Design review of the part built by this model. Coordinates are the model's own, in mm. A direction names the side the tool comes from. Coordinates: 2 decimals unless noted, no trailing zeros. Loops run counter-clockwise (first coordinate to the right, second up) from the corner with the lowest first, then second, coordinate; pieces in that order, holes last. Notation, with made-up numbers: (69, 50.5) -> (126, 50.5) arc R23 ccw to (126, 82.5) -> close; hole circle Ø10 at (27.5, 32.25). An arc over 180 degrees is marked (long way). Answer as a JSON object with one key per item and string values.
```python
from build123d import *

# Parameters (mm, degrees)
SKETCH2_W           = 33.5
SKETCH2_H           = 26
BOSS_EXTRUDE2_DEPTH = 5
FILLET2_R           = 5


with BuildPart() as part:
    # Sketch2 → Boss-Extrude2 (new body)
    # profile 1 of 4: a face of its own
    with BuildSketch(Plane.XY):
        Polygon((-19, -37.5), (-19, -63.5), (-5, -63.5), (-5, -58.5), (5, -58.5), (5, -63.5), (19, -63.5), (19, 63.5), (5, 63.5), (5, 58.5), (-5, 58.5), (-5, 63.5), (-19, 63.5), (-19, 37.5), (-52.5, 37.5), (-52.5, 32.5), (-67.5, 32.5), (-67.5, 37.5), (-75, 37.5), (-75, 0), (-75, -37.5), (-67.5, -37.5), (-67.5, -32.5), (-52.5, -32.5), (-52.5, -37.5), align=None)
    # profile 2 of 4: a face of its own
    with BuildSketch(Plane.XY):
        with Locations((-35.75, 50.5)):
            Rectangle(SKETCH2_W, SKETCH2_H)
        with BuildLine():
            Line((-44.75, 53.5), (-26.75, 53.5))
            ThreePointArc((-26.75, 53.5), (-20.75, 47.5), (-26.75, 41.5))
            Line((-26.75, 41.5), (-44.75, 41.5))
            ThreePointArc((-44.75, 41.5), (-50.75, 47.5), (-44.75, 53.5))
        make_face(mode=Mode.SUBTRACT)
    # profile 3 of 4: a face of its own
    with BuildSketch(Plane.XY):
        with Locations((-35.75, -50.5)):
            Rectangle(SKETCH2_W, SKETCH2_H)
        with BuildLine():
            ThreePointArc((-26.75, -53.5), (-20.75, -47.5), (-26.75, -41.5))
            Line((-26.75, -41.5), (-44.75, -41.5))
            ThreePointArc((-44.75, -41.5), (-50.75, -47.5), (-44.75, -53.5))
            Line((-44.75, -53.5), (-26.75, -53.5))
        make_face(mode=Mode.SUBTRACT)
    # profile 4 of 4: a face of its own
    with BuildSketch(Plane.XY):
        Polygon((-19, -37.5), (-19, -63.5), (-5, -63.5), (-5, -58.5), (5, -58.5), (5, -63.5), (19, -63.5), (19, 63.5), (5, 63.5), (5, 58.5), (-5, 58.5), (-5, 63.5), (-19, 63.5), (-19, 37.5), (-52.5, 37.5), (-52.5, 32.5), (-67.5, 32.5), (-67.5, 37.5), (-75, 37.5), (-75, 0), (-75, -37.5), (-67.5, -37.5), (-67.5, -32.5), (-52.5, -32.5), (-52.5, -37.5), align=None)
    extrude(amount=BOSS_EXTRUDE2_DEPTH)

    # Fillet2
    fillet2_edges = [part.edges().sort_by_distance(p)[0] for p in [
        (19, 63.5, 2.5),
        (19, -63.5, 2.5),
        (-52.5, -63.5, 2.5),
        (-75, -37.5, 2.5),
        (-75, 37.5, 2.5),
        (-52.5, 63.5, 2.5),
    ]]
    fillet(fillet2_edges, radius=FILLET2_R)


solid = part.part
```
1) The part is to be moulded in two halves that separate along Y. For faces 5 (the flat face through (0, 58.5, 2)), 6 (the cylindrical face through (-50.75, -47.37, 2.46)), 7 (the flat face through (19, -1, 2)), say which applies: pulls with the +Y half, pulls with the -Y half, needs draft (parallel to the pull), parting line crosses it, or undercut.
Completed:
{"face 5": "pulls with the +Y half", "face 6": "undercut", "face 7": "needs draft"}
2) Add section B-B, the plane y = 47.5. Give the boundary of the cut face in (x, z), and give its area (4 significant figures).
Completed:
{"outline": "(-52.5, 0) -> (-50.75, 0) -> (-50.75, 5) -> (-52.5, 5) -> close; (-20.75, 0) -> (19, 0) -> (19, 5) -> (-20.75, 5) -> close", "area": "207.5 mm²"}
3) For faces 1 (the flat face through (-67.5, -35, 2)), 2 (the flat face through (-36, 53.5, 2)), 3 (the flat face through (5, 61, 2)), 4 (the flat face through (-69, 37.5, 2)), list the 3-axis set-ups (+Z, -Z, +X, -X, +Y, -Y) from which the entire face can be reached by the end or side of a thin tool; tool diameter is ignored.
Completed:
{"face 1": "+Z, -Z, -Y", "face 2": "+Z, -Z", "face 3": "+Z, -Z, +Y", "face 4": "+Z, -Z, -X, +Y"}
4) Add section C-C, the plane z = 1.65. Count the separate pieces of the cut face and the enclosed holes in it, and give its area (3 significant figures).
Completed:
{"separate pieces": "1", "enclosed holes": "2", "area": "9,830 mm²"}
5) Add section A-A, the plane x = -42. Give the boundary of the cut face in (y, z).
Completed:
{"outline": "(-63.5, 0) -> (-53.5, 0) -> (-53.5, 5) -> (-63.5, 5) -> close; (-41.5, 0) -> (41.5, 0) -> (41.5, 5) -> (-41.5, 5) -> close; (53.5, 0) -> (63.5, 0) -> (63.5, 5) -> (53.5, 5) -> close"}
6) Wall thickness on probe 1 along Y at (x, z) = (-34, 4.1); probe 2 along X at (y, z) = (-48, 0.35); probe 3 along Y at (x, z) = (-24.5, 2.4): over which ranges is each line inside the solid? List them lowest first.
Completed:
{"probe 1": "-63.5 to -53.5, -41.5 to 41.5, 53.5 to 63.5", "probe 2": "-52.5 to -50.73, -20.77 to 19", "probe 3": "-63.5 to -53.06, -41.94 to 41.94, 53.06 to 63.5"}
7) Clearance check with flat-ended pins moving along their axes: pin 1 Ø2 at (y, z) = (-41.5, 3.5) entering from -X; pin 2 Ø2.5 at (x, z) = (0.5, 3.5) entering from -Y; pin 3 Ø0.8 at (x, z) = (-69, 3) entering from +Y. State where each tip first meets the part, or that it passes through.
Completed:
{"pin 1": "x = -52.5", "pin 2": "y = -58.5", "pin 3": "y = 37.5"}
8) Add section D-D, the plane x = -60. Give the boundary of the cut face in (y, z), and give its area (3 significant figures).
Completed:
{"outline": "(-32.5, 0) -> (32.5, 0) -> (32.5, 5) -> (-32.5, 5) -> close", "area": "325 mm²"}
